from build123d import *

# Parameters (mm, degrees)
F0_W       = 152.4
F0_H       = 25.4
F1_DEPTH   = 25.4
F2_W       = 25.4
F2_H       = 16.7976804078
F4_DEPTH   = 3.4544
F5_W       = 25.4
F5_H       = 12.7
F6_DEPTH   = 25.4
F8_W       = 29.1976537555
F8_H       = 3.2747276127
F9_DEPTH   = 25.4
F10_R      = 9.3821167461
F7_R       = 9.84758
F11_DEPTH  = 17.78
F12_R      = 10.1290006818
F12_R_2    = 9.84758
F11_FACE_R = 9.84758
F13_DEPTH  = 0.508
F14_W      = 5.08
F14_H      = 5.08
F15_DEPTH  = 12.7
F16_W      = 5.0729980469
F16_H      = 1.2744938934
F17_DEPTH  = 12.7


with BuildPart() as f1:
    # F0 (on Top) → F1 (new body)
    with BuildSketch(Plane.XY):
        Rectangle(F0_W, F0_H)
    extrude(amount=F1_DEPTH)

    # F2 (on face) → F4 (join)
    with BuildSketch(Plane.YZ.offset(76.2)):
        with Locations((0, 8.3988402039)):
            Rectangle(F2_W, F2_H)
    extrude(amount=-F4_DEPTH)

    # F5 (on face) → F6 (cut)
    with BuildSketch(Plane.YZ.offset(76.2)):
        with Locations((0, 6.35)):
            Rectangle(F5_W, F5_H)
    extrude(amount=-F6_DEPTH, mode=Mode.SUBTRACT)

    # F8 (on face) → F9 (cut)
    with BuildSketch(Plane.XZ.offset(12.7)):
        with Locations((-42.9124059156, 19.2979779094)):
            Rectangle(F8_W, F8_H)
    extrude(amount=-F9_DEPTH, mode=Mode.SUBTRACT)

    # F10
    f10_edges = [f1.edges().sort_by_distance(p)[0] for p in [
        (76.2, -12.7, 19.05),
    ]]
    fillet(f10_edges, radius=F10_R)

    # F7 (on face) → F11 (join)
    with BuildSketch(Plane(origin=(0, 0, 12.7), x_dir=(1, 0, 0), z_dir=(0, 0, -1))):
        with Locations((62.6917358843, 0)):
            Circle(F7_R)
    extrude(amount=F11_DEPTH)

    # F12 (on face) + F11_face (on face) → F13 (join)
    with BuildSketch(Plane(origin=(0, 0, -5.08), x_dir=(1, 0, 0), z_dir=(0, 0, -1))):
        with Locations((62.6917358843, 0)):
            Circle(F12_R)
        with Locations((62.6917358843, 0)):
            Circle(F12_R_2, mode=Mode.SUBTRACT)
        with Locations((62.6917358843, 0)):
            Circle(F12_R_2)
    with BuildSketch(Plane(origin=(62.6917358843, 0, -5.08), x_dir=(1, 0, 0), z_dir=(0, 0, -1))):
        Circle(F11_FACE_R)
    extrude(amount=F13_DEPTH)

    # F14 (on face) → F15 (cut)
    with BuildSketch(Plane(origin=(-76.2, 0, 0), x_dir=(0, -1, 0), z_dir=(-1, 0, 0))):
        with Locations((0, 12.7)):
            Rectangle(F14_W, F14_H)
    extrude(amount=-F15_DEPTH, mode=Mode.SUBTRACT)

    # F16 (on face) → F17 (cut)
    with BuildSketch(Plane.XZ.offset(-2.54)):
        with Locations((-66.0364990234, 14.6027530533)):
            Rectangle(F16_W, F16_H)
    extrude(amount=-F17_DEPTH, mode=Mode.SUBTRACT)


solid = f1.part
Verification items for the finished model (mm, model axes). A direction names the side the tool comes from. Give positions to 0.01 mm unless a question says otherwise; leave off trailing zeros. Write each loop counter-clockwise with the first axis right and the second up, starting at its lowest first coordinate (ties: lowest second). Pieces come first, ordered by that corner, then holes.
(1) Mould release check, pull along Y, two halves, no side actions. Record for faces 1 (the face through (-63.5, 2, 13)), 2 (the face through (-70, 0, 10.16)), 3 (the face through (-43, 0, 17.661)), 4 (the face through (-6, -12.7, 13)): +Y half, -Y half, draft (parallel to the pull), parting line (faces both ways), or undercut.
(2) Material ranges on line 1 (X direction, y = 9.25, z = 20); line 2 (Z direction, x = -33, y = -7); line 3 (Z direction, x = 18, y = 9.25), recorded low to high.
(3) Cross-section at D-D (y = -7.5). Enter the section's corners in (x, z).
(4) Gauge pin test, flat ends, axial feed: pin 1 (4 mm diameter, centred on y = -6, z = 7, fed in from +X); pin 2 (6.5 mm diameter, centred on x = -67.5, y = 2.5, fed in from -Z). Record the tip position at first contact, or that the pin passes through.
(5) Cross-section at A-A (y = 0). Enter the section's corners in (x, z), plus the area to 3 significant figures.
(6) Cross-section at B-B (y = 8.5). Enter the section's corners in (x, z), plus the area to 3 significant figures.
(7) Access from +Z, -Z, +X, -X, +Y, -Y to the whole of each face (thin tool, end or side, straight path). Record for faces 5 (the face through (-70, 2.54, 13)), 6 (the face through (-57.511, 0, 19)), 7 (the face through (-14, 0, 0)).
(8) Cross-section at C-C (x = 2). Enter the section's corners in (y, z).
Worked out:
1. face 1: undercut
1. face 2: undercut
1. face 3: draft
1. face 4: -Y half
2. line 1: x = -76.2 to -57.51, -28.31 to 76.2
2. line 2: z = 0 to 17.66, 20.94 to 25.4
2. line 3: z = 0 to 25.4
3. outline: (-76.2, 0) - (50.8, 0) - (50.8, 12.7) - (56.31, 12.7) - (56.31, -5.08) - (55.88, -5.08) - (55.88, -5.59) - (69.5, -5.59) - (69.5, -5.08) - (69.07, -5.08) - (69.07, 12.7) - (75.22, 12.7) - (75.22, 25.4) - (-76.2, 25.4) - close; hole (-57.51, 17.66) - (-28.31, 17.66) - (-28.31, 20.94) - (-57.51, 20.94) - close
4. pin 1: stops at x = 71.69
4. pin 2: stops at z = 0
5. outline: (-76.2, 0) - (50.8, 0) - (50.8, 12.7) - (52.84, 12.7) - (52.84, -5.08) - (52.56, -5.08) - (52.56, -5.59) - (72.82, -5.59) - (72.82, -5.08) - (72.54, -5.08) - (72.54, 12.7) - (76.2, 12.7) - (76.2, 25.4) - (-76.2, 25.4) - (-76.2, 15.24) - (-63.5, 15.24) - (-63.5, 10.16) - (-76.2, 10.16) - close; hole (-57.51, 17.66) - (-28.31, 17.66) - (-28.31, 20.94) - (-57.51, 20.94) - close
5. area: 3,750 mm2
6. outline: (-76.2, 0) - (50.8, 0) - (50.8, 12.7) - (57.72, 12.7) - (57.72, -5.08) - (57.18, -5.08) - (57.18, -5.59) - (68.2, -5.59) - (68.2, -5.08) - (67.66, -5.08) - (67.66, 12.7) - (76.2, 12.7) - (76.2, 25.4) - (-76.2, 25.4) - close; hole (-68.57, 13.97) - (-63.5, 13.97) - (-63.5, 15.24) - (-68.57, 15.24) - close; hole (-57.51, 17.66) - (-28.31, 17.66) - (-28.31, 20.94) - (-57.51, 20.94) - close
6. area: 3,630 mm2
7. face 5: -X
7. face 6: +Y, -Y
7. face 7: -Z, -X, +Y, -Y
8. outline: (-12.7, 0) - (12.7, 0) - (12.7, 25.4) - (-12.7, 25.4) - close
